from build123d import *

# Parameters (mm, degrees)
F0_R     = 12.7
F0_R_2   = 11.43
F1_DEPTH = 19.05
F2_R     = 12.744954
F3_DEPTH = 1.27


with BuildPart() as f1:
    # F0 (on Top) → F1 (new body)
    with BuildSketch(Plane.XY):
        Circle(F0_R)
        Circle(F0_R_2, mode=Mode.SUBTRACT)
    extrude(amount=F1_DEPTH)

    # F2 (on face) → F3 (join)
    with BuildSketch(Plane(origin=(0, 0, 0), x_dir=(1, 0, 0), z_dir=(0, 0, -1))):
        Circle(F2_R)
    extrude(amount=F3_DEPTH)


solid = f1.part
The model under review builds one solid part; all positions refer to its coordinate system, in mm. Give positions to 0.01 mm unless a question says otherwise; leave off trailing zeros. Write each loop counter-clockwise with the first axis right and the second up, starting at its lowest first coordinate (ties: lowest second). Pieces come first, ordered by that corner, then holes.
1. Wall thickness on L1, parallel to Y at x = 0, z = 7.25; L2, parallel to Z at x = 3.5, y = -8.25; L3, parallel to X at y = -1.25, z = 6.5: over which ranges is each line inside the solid? List them lowest first.
2. Add section B-B, the plane y = 0. Write out the cut boundary in (x, z), plus the area to 3 significant figures.
3. Add section A-A, the plane z = 0.5. Write out the cut boundary in (x, y).
4. Draft analysis for pull direction Y (two halves, no side actions). For faces 1 (the cylindrical face through (-2.763, 12.442, -0.626)), 2 (the cylindrical face through (10.902, 3.433, 9.392)), 3 (the flat face through (0, 0, -1.27)), state which applies: +Y half, -Y half, draft (parallel to the pull), parting line (faces both ways), or undercut.
5. For P1, Ø2, axis at x = 8, z = 6.5, coming from the +Y side; P2, Ø7.5, axis at x = 6, y = -3, coming from the +Z side; P3, Ø3, axis at y = 6.5, z = 9.5, coming from the -X side, all flat-tipped, find the tip position at first contact; note any pin that passes through.
Worked answers:
1. L1: y = -12.7 to -11.43, 11.43 to 12.7
1. L2: z = -1.27 to 0
1. L3: x = -12.64 to -11.36, 11.36 to 12.64
2. outline: (-12.74, -1.27) - (12.74, -1.27) - (12.74, 0) - (12.7, 0) - (12.7, 19.05) - (11.43, 19.05) - (11.43, 0) - (-11.43, 0) - (-11.43, 19.05) - (-12.7, 19.05) - (-12.7, 0) - (-12.74, 0) - close
2. area: 80.8 mm2
3. outline: circle Ø25.4 at (0, 0); hole circle Ø22.86 at (0, 0)
4. face 1: parting line
4. face 2: undercut
4. face 3: draft
5. P1: stops at y = 10.6
5. P2: stops at z = 0
5. P3: stops at x = -11.67
